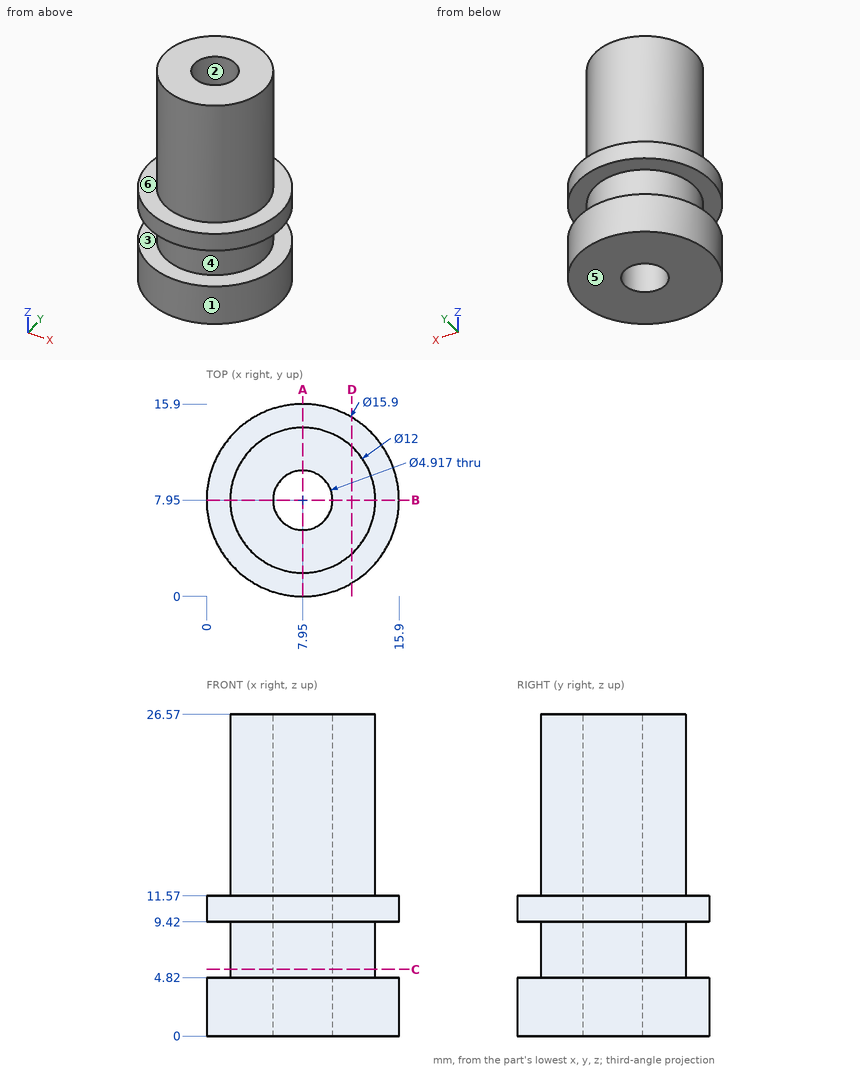
Job drawing, mm, ordinate dimensions from the low corner. One solid piece. A direction names the side the tool comes from. Round coordinates to 2 decimals unless told otherwise and drop trailing zeros. Loops run counter-clockwise (first coordinate to the right, second up) from the corner with the lowest first, then second, coordinate; pieces in that order, holes last.
(1) Two-plate mould, pull along X, no slides. Class the marked faces 1, 2 and 3: +X half, -X half, draft (parallel to the pull), parting line (faces both ways), or undercut.
(2) Which spindle directions (+Z, -Z, +X, -X, +Y, -Y) get a long thin tool onto all of the face, cutting with end or side? Do the marked faces 4, 5 and 6. Say none if no direction does.
(3) Drop flat-ended pins along their axis: pin 1 (8 mm diameter, centred on y = 1.5, z = 22, fed in from +X); pin 2 (5 mm diameter, centred on x = 1.5, z = 12.5, fed in from +Y); pin 3 (1 mm diameter, centred on y = 10, z = 5, fed in from +X). Give the stop position or say it passes through.
(4) Cut at C-C (z = 5.5). Give the cut face in (x, y), plus the area to 3 significant figures.
(5) Cut at D-D (x = 12). Give the cut face in (y, z).
(6) Cut at A-A (x = 7.95). Give the cut face in (y, z).
(7) Wall check: line 1 along Y through (x, z) = (7.95, 11.5); line 2 along Y through (x, z) = (7.95, 5.5); line 3 along Z through (x, y) = (7.25, 1.75). Give the ranges that are in metal, low to high.
Findings below:
1. face 1: parting line
1. face 2: undercut
1. face 3: draft
2. face 4: none
2. face 5: -Z, +X, -X, +Y, -Y
2. face 6: +Z
3. pin 1: stops at x = 13.43
3. pin 2: stops at y = 14.74
3. pin 3: stops at x = 15.74
4. outline: circle Ø12 at (7.95, 7.95); hole circle Ø4.92 at (7.95, 7.95)
4. area: 94.1 mm2
5. outline: (1.11, 0) - (14.79, 0) - (14.79, 4.82) - (12.38, 4.82) - (12.38, 9.42) - (14.79, 9.42) - (14.79, 11.57) - (12.38, 11.57) - (12.38, 26.57) - (3.52, 26.57) - (3.52, 11.57) - (1.11, 11.57) - (1.11, 9.42) - (3.52, 9.42) - (3.52, 4.82) - (1.11, 4.82) - close
6. outline: (0, 0) - (5.49, 0) - (5.49, 26.57) - (1.95, 26.57) - (1.95, 11.57) - (0, 11.57) - (0, 9.42) - (1.95, 9.42) - (1.95, 4.82) - (0, 4.82) - close; (10.41, 0) - (15.9, 0) - (15.9, 4.82) - (13.95, 4.82) - (13.95, 9.42) - (15.9, 9.42) - (15.9, 11.57) - (13.95, 11.57) - (13.95, 26.57) - (10.41, 26.57) - close
7. line 1: y = 0 to 5.49, 10.41 to 15.9
7. line 2: y = 1.95 to 5.49, 10.41 to 13.95
7. line 3: z = 0 to 4.82, 9.42 to 11.57
